For this review, use the dimensioned drawing (mm, ordinates from the lowest corner) and the shaded views. Give positions to 0.01 mm unless a question says otherwise; leave off trailing zeros. Loops run counter-clockwise (first coordinate to the right, second up) from the corner with the lowest first, then second, coordinate; pieces in that order, holes last. Notation, with made-up numbers: M 70,-23 L 92,-23 A8 cw 92,-8 Z; hole C -11,36 d1. An arc over 180 degrees is marked long. Use CSV: the item, a comma, the result in double quotes.
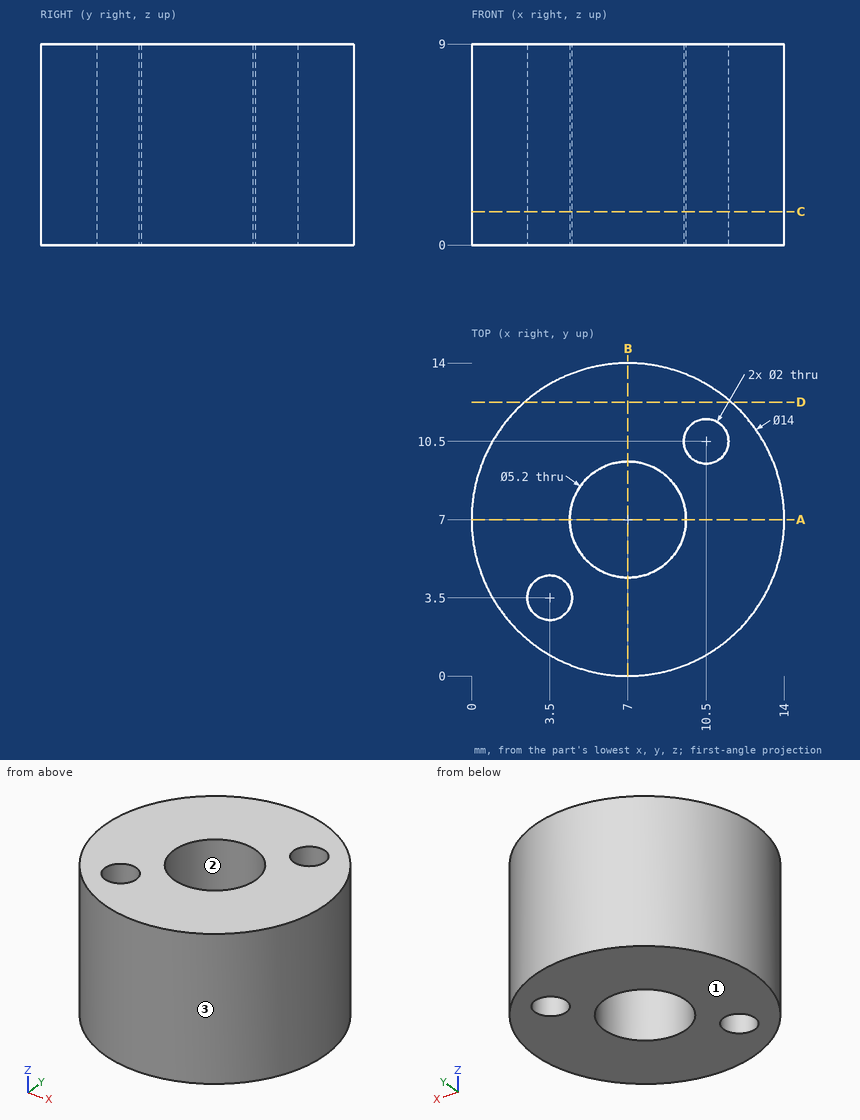
(1) Clearance check with flat-ended pins moving along their axes: P1, Ø2, axis at x = 11.5, z = 1.5, coming from the -Y side; P2, Ø2, axis at y = 12.5, z = 6.5, coming from the -X side; P3, Ø1, axis at x = 9.5, z = 6, coming from the -Y side. State where each tip first meets the part, or that it passes through.
A:
P1,"y = 0.94"
P2,"x = 1.64"
P3,"y = 0.29"
(2) The part is to be moulded in two halves that separate along X. For the marked faces 1, 2 and 3, say which applies: released by +X, released by -X, zero draft, split by the parting line, or undercut.
A:
face 1,"zero draft"
face 2,"undercut"
face 3,"split by the parting line"
(3) We need section D-D on y = 12.25. State the section outline as (x, z) points.
A:
outline,"M 2.37,0 L 11.63,0 L 11.63,9 L 2.37,9 Z"
(4) We need section A-A on y = 7. State the section outline as (x, z) points.
A:
outline,"M 0,0 L 4.4,0 L 4.4,9 L 0,9 Z; M 9.6,0 L 14,0 L 14,9 L 9.6,9 Z"
(5) We need section C-C on z = 1.5. State the section outline as (x, y) points.
A:
outline,"C 7,7 d14; hole C 3.5,3.5 d2; hole C 7,7 d5.2; hole C 10.5,10.5 d2"
(6) Wall thickness on line 1 along Y through (x, z) = (7, 5.5); line 2 along X through (y, z) = (9, 4.25); line 3 along Y through (x, z) = (9.75, 6): over which ranges is each line inside the solid? List them lowest first. Write a range as [from, to].
A:
line 1,"[0, 4.4], [9.6, 14]"
line 2,"[0.29, 5.34], [8.66, 13.71]"
line 3,"[0.56, 9.84], [11.16, 13.44]"
